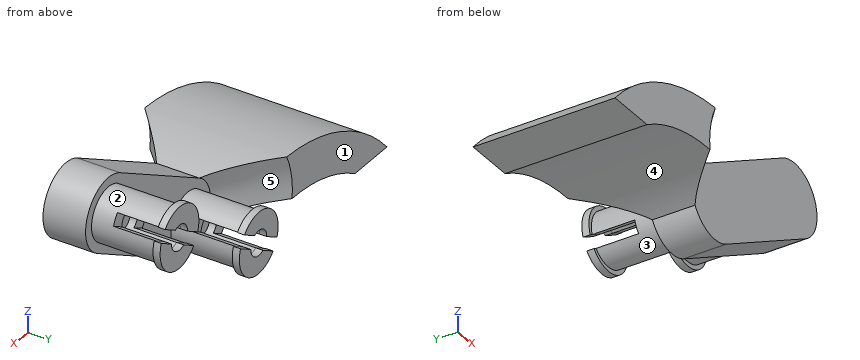
```python
from build123d import *

# Parameters (mm, degrees)
BOSS_EXTRUDE1_DEPTH      = 6
BOSS_EXTRUDE2_DEPTH      = 13
BOSS_EXTRUDE2_DEPTH_BACK = 7
SKETCH1_5_R              = 3.7
SKETCH1_5_R_2            = 1.75
BOSS_EXTRUDE3_DEPTH      = 15
CHAMFER2_SIZE            = 7
CUT_EXTRUDE1_START       = -6
CUT_EXTRUDE1_DEPTH       = 6
SKETCH4_R                = 1.75
BOSS_EXTRUDE5_DEPTH      = 2
BOSS_EXTRUDE6_DEPTH      = 1


with BuildPart() as part:
    # Sketch1 → Boss-Extrude1 (new body)
    with BuildSketch(Plane(origin=(0, 0, 0), x_dir=(1, 0, 0), z_dir=(0, 1, 0))):
        with BuildLine():
            Line((-19.820508076, 5.669872981), (-2.5, -4.330127019))
            ThreePointArc((-2.5, -4.330127019), (4.330127019, -2.5), (2.5, 4.330127019))
            Line((2.5, 4.330127019), (-14.820508076, 14.330127019))
            ThreePointArc((-14.820508076, 14.330127019), (-14.879132605, 14.36276697), (-14.937615699, 14.395659668))
            ThreePointArc((-14.937615699, 14.395659668), (-21.683794323, 12.441666055), (-19.820508076, 5.669872981))
        make_face()
    extrude(amount=BOSS_EXTRUDE1_DEPTH)

    # Sketch1<4> → Boss-Extrude2 (add, two sides: drawn at the far end of the back side and taken through both)
    with BuildSketch(Plane(origin=(0, 0, 0), x_dir=(1, 0, 0), z_dir=(0, 1, 0)).offset(-BOSS_EXTRUDE2_DEPTH_BACK)):
        with BuildLine():
            ThreePointArc((-50, 15), (-36.237721473, 6.041072894), (-19.820508076, 5.669872981))
            ThreePointArc((-19.820508076, 5.669872981), (-22.150137207, 8.705904774), (-21.650635095, 12.5))
            ThreePointArc((-21.650635095, 12.5), (-32.607722458, 11.338333803), (-43, 15))
            Line((-43, 15), (-50, 15))
        make_face()
    extrude(amount=BOSS_EXTRUDE2_DEPTH + BOSS_EXTRUDE2_DEPTH_BACK)

    # Sketch1<5> → Boss-Extrude3 (add)
    # profile 1 of 5: a face of its own
    with BuildSketch(Plane(origin=(0, 0, 0), x_dir=(1, 0, 0), z_dir=(0, 1, 0))):
        with Locations(Location((0, 0, 0), (0, 0, 270))):
            Circle(SKETCH1_5_R)
        with Locations(Location((0, 0, 0), (0, 0, 270))):
            Circle(SKETCH1_5_R_2, mode=Mode.SUBTRACT)
    # profile 2 of 5: a face of its own
    with BuildSketch(Plane(origin=(0, 0, 0), x_dir=(1, 0, 0), z_dir=(0, 1, 0))):
        with BuildLine():
            ThreePointArc((-15.470508076, 13.204293994), (-20.52480207, 11.85), (-19.170508076, 6.795706006))
            Line((-19.170508076, 6.795706006), (-18.195508076, 8.484455543))
            ThreePointArc((-18.195508076, 8.484455543), (-18.836052532, 10.875), (-16.445508076, 11.515544457))
            Line((-16.445508076, 11.515544457), (-15.470508076, 13.204293994))
        make_face()
    # profile 3 of 5: a face of its own
    with BuildSketch(Plane(origin=(0, 0, 0), x_dir=(1, 0, 0), z_dir=(0, 1, 0))):
        with BuildLine():
            Line((-18.195508076, 8.484455543), (-19.170508076, 6.795706006))
            ThreePointArc((-19.170508076, 6.795706006), (-15.470508076, 6.795706006), (-13.620508076, 10))
            ThreePointArc((-13.620508076, 10), (-14.116214082, 11.85), (-15.470508076, 13.204293994))
            Line((-15.470508076, 13.204293994), (-16.445508076, 11.515544457))
            ThreePointArc((-16.445508076, 11.515544457), (-15.804963619, 10.875), (-15.570508076, 10))
            ThreePointArc((-15.570508076, 10), (-16.445508076, 8.484455543), (-18.195508076, 8.484455543))
        make_face()
    # profile 4 of 5: a face of its own
    with BuildSketch(Plane(origin=(0, 0, 0), x_dir=(1, 0, 0), z_dir=(0, 1, 0))):
        with BuildLine():
            ThreePointArc((-15.470508076, 13.204293994), (-20.52480207, 11.85), (-19.170508076, 6.795706006))
            Line((-19.170508076, 6.795706006), (-18.195508076, 8.484455543))
            ThreePointArc((-18.195508076, 8.484455543), (-18.836052532, 10.875), (-16.445508076, 11.515544457))
            Line((-16.445508076, 11.515544457), (-15.470508076, 13.204293994))
        make_face()
    # profile 5 of 5: a face of its own
    with BuildSketch(Plane(origin=(0, 0, 0), x_dir=(1, 0, 0), z_dir=(0, 1, 0))):
        with BuildLine():
            Line((-18.195508076, 8.484455543), (-19.170508076, 6.795706006))
            ThreePointArc((-19.170508076, 6.795706006), (-15.470508076, 6.795706006), (-13.620508076, 10))
            ThreePointArc((-13.620508076, 10), (-14.116214082, 11.85), (-15.470508076, 13.204293994))
            Line((-15.470508076, 13.204293994), (-16.445508076, 11.515544457))
            ThreePointArc((-16.445508076, 11.515544457), (-15.804963619, 10.875), (-15.570508076, 10))
            ThreePointArc((-15.570508076, 10), (-16.445508076, 8.484455543), (-18.195508076, 8.484455543))
        make_face()
    extrude(amount=BOSS_EXTRUDE3_DEPTH)

    # Chamfer2
    chamfer2_edges = [part.edges().sort_by_distance(p)[0] for p in [
        (-22.150137207, -7, -8.705904774),
        (-22.150137207, 13, -8.705904774),
    ]]
    chamfer(chamfer2_edges, length=CHAMFER2_SIZE - 0.0001)  # a hair under: the kernel refuses the full size

    # Sketch3 → Cut-Extrude1 (cut)
    with BuildSketch(Plane(origin=(0, 15, 0), x_dir=(1, 0, 0), z_dir=(0, 1, 0)).offset(CUT_EXTRUDE1_START)):
        with BuildLine():
            Line((-20.014101509, 12.536642351), (-18.220272206, 11.50097452))
            ThreePointArc((-18.220272206, 11.50097452), (-18.836052532, 10.875), (-19.070272206, 10.028731334))
            Line((-19.070272206, 10.028731334), (-20.864101509, 11.064399165))
            ThreePointArc((-20.864101509, 11.064399165), (-20.52480207, 11.85), (-20.014101509, 12.536642351))
        make_face()
        with BuildLine():
            Line((-13.776914643, 8.935600835), (-15.570743946, 9.971268666))
            ThreePointArc((-15.570743946, 9.971268666), (-15.804963619, 9.125), (-16.420743946, 8.49902548))
            Line((-16.420743946, 8.49902548), (-14.626914643, 7.463357649))
            ThreePointArc((-14.626914643, 7.463357649), (-14.116214082, 8.15), (-13.776914643, 8.935600835))
        make_face()
        with BuildLine():
            Line((2.693593433, -2.536642351), (0.89976413, -1.50097452))
            ThreePointArc((0.89976413, -1.50097452), (1.515544457, -0.875), (1.74976413, -0.028731334))
            Line((1.74976413, -0.028731334), (3.543593433, -1.064399165))
            ThreePointArc((3.543593433, -1.064399165), (3.204293994, -1.85), (2.693593433, -2.536642351))
        make_face()
        with BuildLine():
            Line((-3.543593433, 1.064399165), (-1.74976413, 0.028731334))
            ThreePointArc((-1.74976413, 0.028731334), (-1.515544457, 0.875), (-0.89976413, 1.50097452))
            Line((-0.89976413, 1.50097452), (-2.693593433, 2.536642351))
            ThreePointArc((-2.693593433, 2.536642351), (-3.204293994, 1.85), (-3.543593433, 1.064399165))
        make_face()
    extrude(amount=CUT_EXTRUDE1_DEPTH, mode=Mode.SUBTRACT)

    # Sketch4 → Boss-Extrude5 (add)
    with BuildSketch(Plane(origin=(0, 6, 0), x_dir=(1, 0, 0), z_dir=(0, 1, 0))):
        with Locations(Location((-17.320508076, 10, 0), (0, 0, 120.940718932))):
            Circle(SKETCH4_R)
        with Locations(Location((0, 0, 0), (0, 0, 90))):
            Circle(SKETCH4_R)
    extrude(amount=BOSS_EXTRUDE5_DEPTH)

    # Sketch6 → Boss-Extrude6 (add)
    with BuildSketch(Plane(origin=(0, 15, 0), x_dir=(1, 0, 0), z_dir=(0, 1, 0))):
        with BuildLine():
            Line((-18.220272206, 11.50097452), (-20.447114211, 12.786642351))
            ThreePointArc((-20.447114211, 12.786642351), (-15.161973233, 13.738692017), (-13.343901941, 8.685600835))
            Line((-13.343901941, 8.685600835), (-15.570743946, 9.971268666))
            ThreePointArc((-15.570743946, 9.971268666), (-16.445508076, 11.515544457), (-18.220272206, 11.50097452))
        make_face()
        with BuildLine():
            Line((-16.420743946, 8.49902548), (-14.193901941, 7.213357649))
            ThreePointArc((-14.193901941, 7.213357649), (-19.479042918, 6.261307983), (-21.297114211, 11.314399165))
            Line((-21.297114211, 11.314399165), (-19.070272206, 10.028731334))
            ThreePointArc((-19.070272206, 10.028731334), (-18.195508076, 8.484455543), (-16.420743946, 8.49902548))
        make_face()
        with BuildLine():
            Line((0.89976413, -1.50097452), (3.126606135, -2.786642351))
            ThreePointArc((3.126606135, -2.786642351), (-2.158534843, -3.738692017), (-3.976606135, 1.314399165))
            Line((-3.976606135, 1.314399165), (-1.74976413, 0.028731334))
            ThreePointArc((-1.74976413, 0.028731334), (-0.875, -1.515544457), (0.89976413, -1.50097452))
        make_face()
        with BuildLine():
            Line((-0.89976413, 1.50097452), (-3.126606135, 2.786642351))
            ThreePointArc((-3.126606135, 2.786642351), (2.158534843, 3.738692017), (3.976606135, -1.314399165))
            Line((3.976606135, -1.314399165), (1.74976413, -0.028731334))
            ThreePointArc((1.74976413, -0.028731334), (0.875, 1.515544457), (-0.89976413, 1.50097452))
        make_face()
    extrude(amount=BOSS_EXTRUDE6_DEPTH)


solid = part.part
```
Input: part model. Units: mm. Frame: model coordinates. Face numbers are marked on the shaded views. A direction names the side the tool comes from. Round coordinates to 2 decimals unless told otherwise and drop trailing zeros. Loops run counter-clockwise (first coordinate to the right, second up) from the corner with the lowest first, then second, coordinate; pieces in that order, holes last. Notation, with made-up numbers: (2.25, 75.5) -> (17.25, 75.5) arc R18 ccw to (17.25, 105.5) -> close; hole circle Ø8 at (78.25, 35). An arc over 180 degrees is marked (long way). Use one line per item in the form item = value. Start each with the question number.
Item 1: Section query A-A on y = 5. Return the cut outline in (x, z), then the cut area to 3 significant figures.
Item 2: Material intervals for L1, parallel to Z at x = 0, y = 12.75; L2, parallel to Y at x = -20.5, z = -6.75, sorted ascending. Write a range as from..to.
Item 3: Section query D-D on y = -4.25. Return the cut outline in (x, z), then the cut area to 3 significant figures.
Item 4: Set-up query: the marked faces 4 and 5. Return all of +Z, -Z, +X, -X, +Y, -Y with unobstructed straight access to the full face (end or side cutting, diameter ignored); none if empty.
Item 5: Contact query for flat-ended pins moving along their axis: pin 1 Ø4 at (x, z) = (0, 0) entering from -Y; pin 2 Ø11.5 at (x, z) = (-43, -10) entering from +Y; pin 3 Ø10 at (x, z) = (-35, 2) entering from -Y; pin 4 Ø1 at (x, z) = (-17, -11) entering from +Y. Output: stop coordinate, or through.
Item 6: Section query C-C on x = -31.5. Return the cut outline in (y, z).
Item 7: Section query B-B on x = 0. Return the cut outline in (y, z), then the cut area to 3 significant figures.
Item 8: Mould query, pull axis X, two halves, no side actions, for the marked faces 1, 2 and 3. Classes: pulls with the +X half, pulls with the -X half, needs draft (parallel to the pull), parting line crosses it, or undercut.
Ans:
q1.outline = (-50, -15) -> (-43, -15) arc R25 cw to (-21.65, -12.5) arc R5 ccw to (-14.94, -14.4) arc R15.54 cw to (-14.82, -14.33) -> (2.5, -4.33) arc R5 ccw to (-2.5, 4.33) -> (-19.82, -5.67) arc R30 ccw to start
q1.area = 436 mm^2
q2.L1 = -3.7..-1.75, 1.75..3.7
q2.L2 = 0..6
q3.outline = (-50, -15) -> (-43, -15) arc R25 cw to (-26.47, -11.38) arc R9.25 cw to (-24.97, -4.8) arc R30 ccw to start
q3.area = 126 mm^2
q4.face_4 = -Z, +Y, -Y
q4.face_5 = +Y
q5.pin_1 = 0
q5.pin_2 = 13
q5.pin_3 = through
q5.pin_4 = 8
q6.outline = (-7, -11.23) -> (13, -11.23) -> (13, -4.99) -> (-7, -4.99) -> close
q7.outline = (0, -5.77) -> (6, -5.77) -> (6, -3.7) -> (15, -3.7) -> (15, -4.3) -> (16, -4.3) -> (16, -1.75) -> (8, -1.75) -> (8, 1.75) -> (16, 1.75) -> (16, 4.3) -> (15, 4.3) -> (15, 3.7) -> (6, 3.7) -> (6, 5) -> (0, 5) -> close
q7.area = 112 mm^2
q8.face_1 = needs draft
q8.face_2 = parting line crosses it
q8.face_3 = undercut
